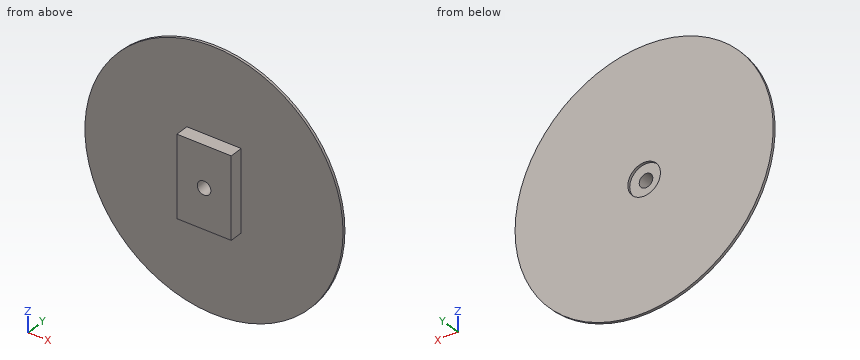
```python
from build123d import *

# Parameters (mm, degrees)
F0_R     = 60.325
F0_R_2   = 7.62
F1_DEPTH = 1.1938
F2_R     = 7.62
F3_DEPTH = 6.35
F4_R     = 3.175
F5_DEPTH = 25.4


with BuildPart() as f1:
    # F0 (on Front) → F1 (new body)
    with BuildSketch(Plane.XZ):
        Circle(F0_R)
        Circle(F0_R_2, mode=Mode.SUBTRACT)
    extrude(amount=F1_DEPTH)

    # F2 (on face) → F3 (join)
    with BuildSketch(Plane.XZ.offset(1.1938)):
        Polygon((12.7, 19.392626), (0, 19.392626), (-12.7, 19.392626), (-12.7, -18.707374), (12.7, -18.707374), align=None)
        Circle(F2_R, mode=Mode.SUBTRACT)
        Circle(F2_R)
    extrude(amount=F3_DEPTH)

    # F4 (on face) → F5 (cut)
    with BuildSketch(Plane.XZ.offset(7.5438)):
        Circle(F4_R)
    extrude(amount=-F5_DEPTH, mode=Mode.SUBTRACT)


solid = f1.part
```
Work out the finished part from the listing and answer in its coordinate system (mm). Coordinates: 2 decimals unless noted, no trailing zeros. Write each loop counter-clockwise with the first axis right and the second up, starting at its lowest first coordinate (ties: lowest second). Pieces come first, ordered by that corner, then holes.
Q1. A cutting plane is placed at A-A, the plane z = 0. Give the vertices of the cut face in (x, y) (3 decimals), then the cut area to 3 significant figures.
Q2. A cutting plane is placed at D-D, the plane z = 17.5. Give the vertices of the cut face in (x, y), then the cut area to 3 significant figures.
Q3. A cutting plane is placed at B-B, the plane x = 0. Give the vertices of the cut face in (y, z) (3 decimals).
Q4. Find the intervals of material crossed by line 1 (Z direction, x = 0, y = -0.5) (3 decimals); line 2 (Z direction, x = 0, y = -4) (3 decimals); line 3 (Y direction, x = -47, z = 13), in increasing order.
Q5. Each of these flat-tipped pins is pushed along its axis until it touches: pin 1 Ø4 at (x, y) = (-10, -6.5) entering from -Z; pin 2 Ø4 at (x, y) = (6.5, -2) entering from -Z; pin 3 Ø3 at (y, z) = (-4.5, -2.5) entering from +X; pin 4 Ø1.5 at (x, z) = (8, -48) entering from +Y. Where does it stop, or does it pass through?
Q6. A cutting plane is placed at C-C, the plane y = -2.75. Give the vertices of the cut face in (x, z) (3 decimals), then the cut area to 3 significant figures.
Findings below:
1. outline: (-60.325, -1.194) - (-12.7, -1.194) - (-12.7, -7.544) - (-3.175, -7.544) - (-3.175, -1.194) - (-7.62, -1.194) - (-7.62, 0) - (-60.325, 0) - close; (3.175, -7.544) - (12.7, -7.544) - (12.7, -1.194) - (60.325, -1.194) - (60.325, 0) - (7.62, 0) - (7.62, -1.194) - (3.175, -1.194) - close
1. area: 247 mm2
2. outline: (-57.73, -1.19) - (-12.7, -1.19) - (-12.7, -7.54) - (12.7, -7.54) - (12.7, -1.19) - (57.73, -1.19) - (57.73, 0) - (-57.73, 0) - close
2. area: 299 mm2
3. outline: (-7.544, -18.707) - (-1.194, -18.707) - (-1.194, -60.325) - (0, -60.325) - (0, -7.62) - (-1.194, -7.62) - (-1.194, -3.175) - (-7.544, -3.175) - close; (-7.544, 3.175) - (-1.194, 3.175) - (-1.194, 7.62) - (0, 7.62) - (0, 60.325) - (-1.194, 60.325) - (-1.194, 19.393) - (-7.544, 19.393) - close
4. line 1: z = -60.325 to -7.62, 7.62 to 60.325
4. line 2: z = -18.707 to -3.175, 3.175 to 19.393
4. line 3: y = -1.19 to 0
5. pin 1: stops at z = -18.71
5. pin 2: stops at z = -60.14
5. pin 3: stops at x = 12.7
5. pin 4: stops at y = 0
6. outline: (-12.7, -18.707) - (12.7, -18.707) - (12.7, 19.393) - (-12.7, 19.393) - close; hole circle Ø6.35 at (0, 0)
6. area: 936 mm2
